from build123d import *

# Parameters (mm, degrees)
CHAMFER_1_SIZE      = 2
CUT_EXTRUDE_START   = -11.5
SKETCH_2_W          = 25
SKETCH_2_H          = 4
CUT_EXTRUDE_1_DEPTH = 28


with BuildPart() as part:
    # 草图1 → 旋转1 (revolve)
    with BuildSketch(Plane.XY, mode=Mode.PRIVATE) as revolve_1_sk:
        Polygon((0, 0), (0, 9), (28, 9), (28, 10.5), (80.5, 10.5), (80.5, 12.5), (129.1, 12.5), (129.1, 15), (172.7, 15), (172.7, 16.25), (178.7, 16.25), (178.7, 15), (252.6, 15), (252.6, 12.5), (264.6, 12.5), (264.6, 0), align=None)
    revolve(revolve_1_sk.sketch.rotate(Axis((264.6, 0, 0), (-1, 0, 0)), 90), axis=Axis((264.6, 0, 0), (-1, 0, 0)))

    # 倒角1
    chamfer_1_edges = [part.edges().sort_by_distance(p)[0] for p in [
        (264.6, 0, 12.5),
        (0, 0, 9),
    ]]
    chamfer(chamfer_1_edges, length=CHAMFER_1_SIZE)

    # 草图2 → 切除-拉伸1 (cut)
    with BuildSketch(Plane.XY.offset(CUT_EXTRUDE_START)):
        with Locations((150.9, -2)):
            Rectangle(SKETCH_2_W, SKETCH_2_H)
        with Locations((150.9, 2)):
            Rectangle(SKETCH_2_W, SKETCH_2_H)
    extrude(amount=-CUT_EXTRUDE_1_DEPTH, mode=Mode.SUBTRACT)


solid = part.part
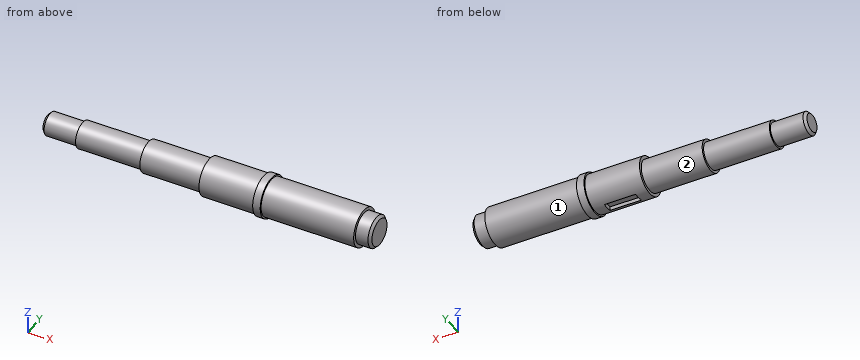
Could you check a few things on this model? Use its own coordinates, in mm. Face numbers are marked on the shaded views. A direction names the side the tool comes from. Coordinates: 2 decimals unless noted, no trailing zeros. Write each loop counter-clockwise with the first axis right and the second up, starting at its lowest first coordinate (ties: lowest second). Pieces come first, ordered by that corner, then holes. Notation, with made-up numbers: (25, -23.5) - (76, -23.5) arc R9 ccw to (76, -16.5) - close; hole circle Ø9 at (14, 76.25). An arc over 180 degrees is marked (long way). Write item = value, one per line.
1) Suppose I cut it at C-C on x = 243. Please give me the cut outline in (y, z).
Result set:
outline = circle Ø30 at (0, 0)
2) Suppose I cut it at D-D on x = 107.5. Please give me the cut outline in (y, z).
Result set:
outline = circle Ø25 at (0, 0)
3) Suppose I cut it at B-B on x = 160. Please give me the cut outline in (y, z), plus the area to 3 significant figures.
Result set:
outline = (-4, -14.46) - (-4, -11.5) - (4, -11.5) - (4, -14.46) arc R15 ccw (long way) to start
area = 680 mm2
4) Please list where these lines run through material, in increasing order: line 1 (Y direction, x = 148.5, z = -0.5); line 2 (X direction, y = -11, z = -6); line 3 (Y direction, x = 230, z = 12). Write a range as [from, to].
Result set:
line_1 = [-14.99, 14.99]
line_2 = [129.1, 252.6]
line_3 = [-9, 9]
5) For the marked faces 1 and 2, which set-ups out of +Z, -Z, +X, -X, +Y, -Y let a thin tool reach every point of the face, with its end or its side?
Result set:
face_1 = +X
face_2 = -X
6) Will these pins go through, and if not, where does the flat tip stop? pin 1 Ø8 at (x, z) = (209.5, 6) entering from +Y; pin 2 Ø10 at (x, z) = (90, 1) entering from +Y; pin 3 Ø2 at (x, y) = (224, 5.5) entering from -Z; pin 4 Ø12 at (y, z) = (-7, 7) entering from -X.
Result set:
pin_1 = 14.87
pin_2 = 12.5
pin_3 = -14.31
pin_4 = 0
